The figure shows three views and two pictorial views of one solid part (mm, origin at its lowest corner). Answer the questions. A direction names the side the tool comes from. Coordinates: 2 decimals unless noted, no trailing zeros. Write each loop counter-clockwise with the first axis right and the second up, starting at its lowest first coordinate (ties: lowest second). Pieces come first, ordered by that corner, then holes.
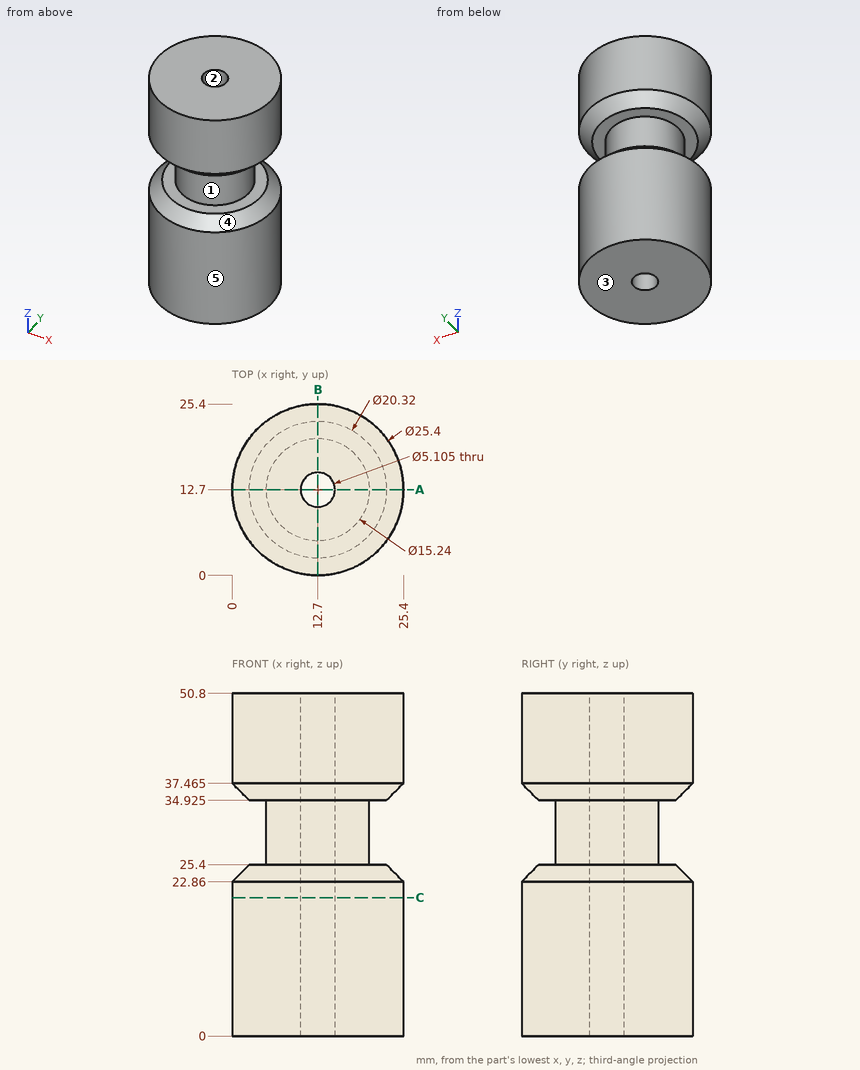
1. Flat-ended cylindrical pins translate along their axes: P1, Ø6, axis at y = 4.5, z = 8.5, coming from the -X side; P2, Ø10, axis at x = 5.5, z = 31.5, coming from the -Y side (1 decimal); P3, Ø4, axis at x = 18.5, z = 35.5, coming from the -Y side. Find the tip coordinate at first contact, or state that the pin passes through.
Results found:
P1: stops at x = 1.11
P2: stops at y = 2.6
P3: stops at y = 1.17
2. Section A-A on y = 12.7 is taken. Give the vertices of the cut face in (x, z) (1 decimal).
Results found:
outline: (0, 0) - (10.1, 0) - (10.1, 50.8) - (0, 50.8) - (0, 37.5) - (2.5, 34.9) - (5.1, 34.9) - (5.1, 25.4) - (2.5, 25.4) - (0, 22.9) - close; (15.3, 0) - (25.4, 0) - (25.4, 22.9) - (22.9, 25.4) - (20.3, 25.4) - (20.3, 34.9) - (22.9, 34.9) - (25.4, 37.5) - (25.4, 50.8) - (15.3, 50.8) - close
3. Find the intervals of material crossed by L1, parallel to Y at x = 12.7, z = 12; L2, parallel to X at y = 12.7, z = 34; L3, parallel to Z at x = 20.25, y = 6.5 (1 decimal), in increasing order.
Results found:
L1: y = 0 to 10.15, 15.25 to 25.4
L2: x = 5.08 to 10.15, 15.25 to 20.32
L3: z = 0 to 25.4, 34.9 to 50.8
4. A tool of negligible diameter and unlimited length cuts with its end or side. For the marked faces 1 and 2, from which of +Z, -Z, +X, -X, +Y, -Y can it reach the whole face along a straight path? Write none if from no direction.
Results found:
face 1: none
face 2: +Z, -Z
5. Section C-C on z = 20.5 is taken. Give the vertices of the cut face in (x, y) (1 decimal).
Results found:
outline: circle Ø25.4 at (12.7, 12.7); hole circle Ø5.1 at (12.7, 12.7)
6. For a pull along Z with two mould halves and no side action, classify the marked faces 3, 4 and 5 as pulls with the +Z half, pulls with the -Z half, needs draft (parallel to the pull), parting line crosses it, or undercut.
Results found:
face 3: pulls with the -Z half
face 4: undercut
face 5: needs draft
